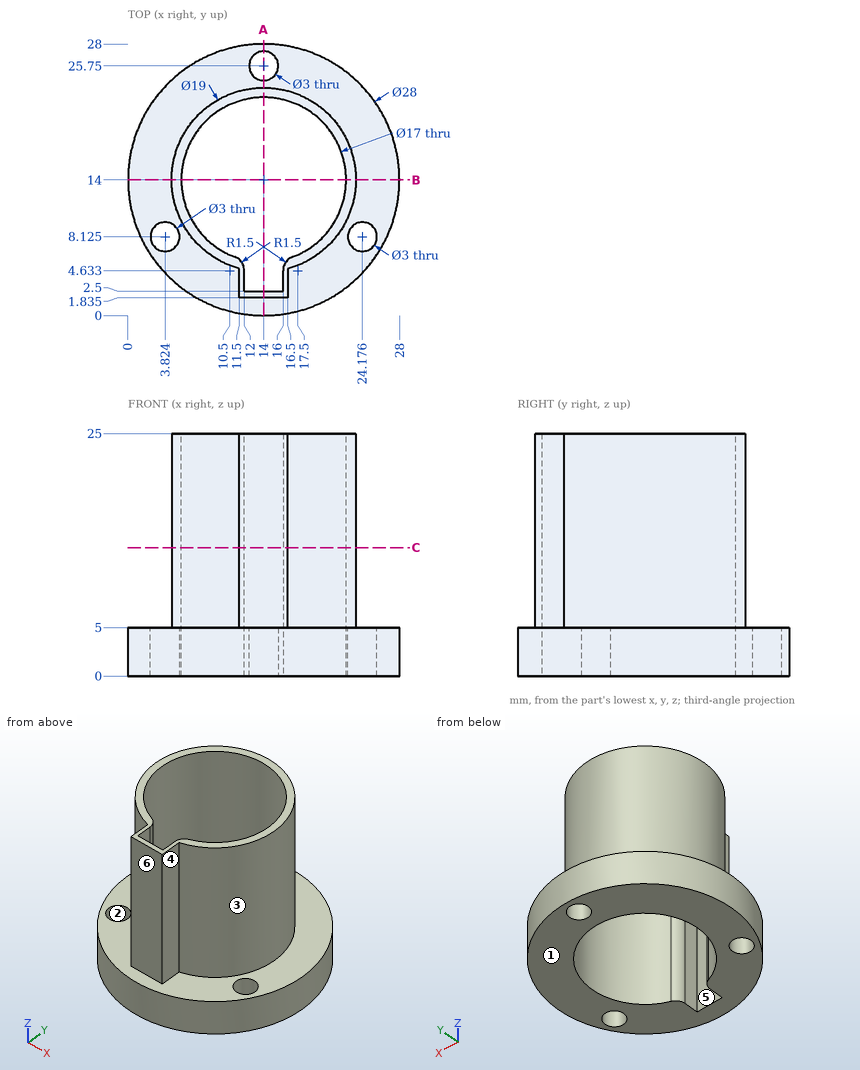
Geometry check sheet. Reference: drawing and pictorial views, mm from the part's lowest x, y, z. A direction names the side the tool comes from. Round coordinates to 2 decimals unless told otherwise and drop trailing zeros. Write each loop counter-clockwise with the first axis right and the second up, starting at its lowest first coordinate (ties: lowest second). Pieces come first, ordered by that corner, then holes. Notation, with made-up numbers: (86, 61) -> (142, 61) arc R22 ccw to (142, 80) -> close; hole circle Ø9 at (-35.5, -27.75). An arc over 180 degrees is marked (long way). Answer as CSV lines item,"result". Start each with the question number.
1) Section check B-B on y = 14. Enter the section's corners in (x, z).
2) Section check C-C on z = 13.25. Enter the section's corners in (x, y) (1 decimal).
3) Release check for a two-part mould opening along Y. For the marked faces 1, 2 and 3 record: pulls with the +Y half, pulls with the -Y half, needs draft (parallel to the pull), parting line crosses it, or undercut.
4) Tool access check on the marked faces 4, 5 and 6. Record the directions out of +Z, -Z, +X, -X, +Y, -Y that give a thin tool (end or side, any length) a straight path to the whole face; none if there is none.
5) Section check A-A on x = 14. State how many separate pieces and enclosed holes the cut face has.
6) Go/stop test with flat-tipped pins: P1, Ø1.5, axis at y = 4, z = 16.5, coming from the -X side; P2, Ø10, axis at x = 14, y = 14, coming from the +Z side; P3, Ø3.5, axis at x = 14, y = 25.75, coming from the +Z side; P4, Ø1.5, axis at x = 24.5, z = 5.5, coming from the -Y side. Record where each tip stops, or that it passes through.
7) Material ranges on line 1 (X direction, y = 2.75, z = 8.5); line 2 (X direction, y = 14, z = 19.25); line 3 (Y direction, x = 15.5, z = 19.75) (1 decimal), recorded low to high. Write a range as from..to.
Found:
1,outline,"(0, 0) -> (5.5, 0) -> (5.5, 25) -> (4.5, 25) -> (4.5, 5) -> (0, 5) -> close; (22.5, 0) -> (28, 0) -> (28, 5) -> (23.5, 5) -> (23.5, 25) -> (22.5, 25) -> close"
2,outline,"(11.5, 1.8) -> (16.5, 1.8) -> (16.5, 4.8) arc R9.5 ccw (long way) to (11.5, 4.8) -> close; hole (11, 6) arc R1.5 cw to (12, 4.6) -> (12, 2.5) -> (16, 2.5) -> (16, 4.6) arc R1.5 cw to (17, 6) arc R8.5 ccw (long way) to start"
3,face 1,"needs draft"
3,face 2,"undercut"
3,face 3,"parting line crosses it"
4,face 4,"+Z, +X, -Y"
4,face 5,"+Z, -Z"
4,face 6,"+Z, +X, -X, -Y"
5,separate pieces,"3"
5,enclosed holes,"0"
6,P1,"stops at x = 11.5"
6,P2,"passes through"
6,P3,"stops at z = 5"
6,P4,"stops at y = 4.14"
7,line 1,"x = 11.5..12, 16..16.5"
7,line 2,"x = 4.5..5.5, 22.5..23.5"
7,line 3,"y = 1.8..2.5, 22.4..23.4"
